from build123d import *

# Parameters (mm, degrees)
PICOVER_DEPTH                       = 40
PICOVER_DEPTH_BACK                  = 2
SKETCH1_W                           = 139.991389113
SKETCH1_H                           = 97.393342316
SKETCH2_W                           = 96.759944342
SKETCH2_H                           = 98.11966003
OPENINGFORPI_DEPTH                  = 37
SKETCH4_W                           = 18
SKETCH4_H                           = 97.393342316
CUTAWAYSTHATDEFINESCREWPLATES_DEPTH = 30
BOSS_EXTRUDE1_DEPTH                 = 97.393342316
HOLEFORPOWERHDMIAUDIO_DEPTH         = 150
HOLEFORPOWERHDMIAUDIO_DEPTH_BACK    = 30
SKETCH6_W                           = 65.470403297
SKETCH6_H                           = 37
SKETCH7_R                           = 2.75
CUT_EXTRUDE7_DEPTH                  = 60
FILLET1_R                           = 30
FILLET2_R                           = 30
FILLET3_R                           = 30
FILLET4_R                           = 30


with BuildPart() as part:
    # Sketch1 → PiCover (new, two sides: drawn at the far end of the back side and taken through both)
    with BuildSketch(Plane(origin=(0, 0, 0), x_dir=(1, 0, 0), z_dir=(0, 1, 0)).offset(-PICOVER_DEPTH_BACK)):
        with Locations((69.995694556, 48.696671158)):
            Rectangle(SKETCH1_W, SKETCH1_H)
    extrude(amount=PICOVER_DEPTH + PICOVER_DEPTH_BACK)

    # Sketch2 → OpeningForPi (cut)
    with BuildSketch(Plane(origin=(0, 40, 0), x_dir=(1, 0, 0), z_dir=(0, 1, 0))):
        with Locations((70.044375284, 48.333512301)):
            Rectangle(SKETCH2_W, SKETCH2_H)
    extrude(amount=-OPENINGFORPI_DEPTH, mode=Mode.SUBTRACT)

    # Sketch4 → CutAwaysThatDefineScrewPlates (cut)
    with BuildSketch(Plane.XZ.offset(2)):
        with Locations((130.991389113, -48.696671158)):
            Rectangle(SKETCH4_W, SKETCH4_H)
        with Locations((9, -48.696671158)):
            Rectangle(SKETCH4_W, SKETCH4_H)
    extrude(amount=-CUTAWAYSTHATDEFINESCREWPLATES_DEPTH, mode=Mode.SUBTRACT)

    # Sketch11 → Boss-Extrude1 (add)
    with BuildSketch(Plane.XY):
        Polygon((0, 28), (18, 28), (18, -2), align=None)
        Polygon((139.991389113, 28), (121.991389113, 28), (121.991389113, -2), align=None)
    extrude(amount=-BOSS_EXTRUDE1_DEPTH)

    # Sketch6 → HoleForPowerHDMIAudio (cut, two sides: drawn at the far end of the back side and taken through both)
    with BuildSketch(Plane(origin=(21.664403113, 0, 0), x_dir=(0, 0, -1), z_dir=(1, 0, 0)).offset(-HOLEFORPOWERHDMIAUDIO_DEPTH_BACK)):
        with Locations((47.655232797, 21.5)):
            Rectangle(SKETCH6_W, SKETCH6_H)
    extrude(amount=HOLEFORPOWERHDMIAUDIO_DEPTH + HOLEFORPOWERHDMIAUDIO_DEPTH_BACK, mode=Mode.SUBTRACT)

    # Sketch7 → Cut-Extrude7 (cut)
    with BuildSketch(Plane(origin=(0, 40, 0), x_dir=(1, 0, 0), z_dir=(0, 1, 0))):
        with Locations(Location((6.934452889, 8.128892452, 0), (0, 0, 270))):
            Circle(SKETCH7_R)
        with Locations(Location((6.934452889, 91.275593332, 0), (0, 0, 270))):
            Circle(SKETCH7_R)
        with Locations(Location((130.288718206, 89.274198859, 0), (0, 0, 270))):
            Circle(SKETCH7_R)
        with Locations(Location((129.818664093, 7.39541328, 0), (0, 0, 270))):
            Circle(SKETCH7_R)
    extrude(amount=-CUT_EXTRUDE7_DEPTH, mode=Mode.SUBTRACT)

    # Fillet1
    fillet1_edges = [part.edges().sort_by_distance(p)[0] for p in [
        (21.664403113, 3, -88.891888381),
    ]]
    fillet(fillet1_edges, radius=FILLET1_R)

    # Fillet2
    fillet2_edges = [part.edges().sort_by_distance(p)[0] for p in [
        (118.424347455, 3, -88.891888381),
    ]]
    fillet(fillet2_edges, radius=FILLET2_R)

    # Fillet3
    fillet3_edges = [part.edges().sort_by_distance(p)[0] for p in [
        (21.664403113, 3, -7.460015574),
    ]]
    fillet(fillet3_edges, radius=FILLET3_R)

    # Fillet4
    fillet4_edges = [part.edges().sort_by_distance(p)[0] for p in [
        (118.424347455, 3, -7.460015574),
    ]]
    fillet(fillet4_edges, radius=FILLET4_R)


solid = part.part
Build history of the part. All positions in model axes, mm. A direction names the side the tool comes from. Round coordinates to 2 decimals unless told otherwise and drop trailing zeros. Write each loop counter-clockwise with the first axis right and the second up, starting at its lowest first coordinate (ties: lowest second). Pieces come first, ordered by that corner, then holes. Notation, with made-up numbers: M 57,15 L 76,15 A21 ccw 76,47 Z; hole C 9.5,-35 d4. An arc over 180 degrees is marked long. Answer as a JSON object with one key per item and string values. Group by question number.
(1) Flat gauge pins, fed straight in: pin 1 (6 mm diameter, centred on y = 26.5, z = -85.5, fed in from -X); pin 2 (1 mm diameter, centred on x = 57, z = -46, fed in from +Y); pin 3 (6.5 mm diameter, centred on x = 129.82, z = -7.4, fed in from -Y); pin 4 (6.5 mm diameter, centred on x = 130.29, z = -89.27, fed in from -Y). Where does each tip first touch, or does it go through?
(2) Drill centre lines: L1, parallel to Z at x = 7, y = 22; L2, parallel to X at y = 32.5, z = -84; L3, parallel to Z at x = 17, y = 24. Where is each one in solid material? Low to high.
(3) Cut at A-A (y = 26). Give the cut face in (x, z).
(4) Mould opens along X. For faces 5 (the flat face through (124.865, 2.79, -48.015)), 6 (the flat face through (127, 40, -89)), 7 (the flat face through (118.424, 37, -89)) say: pulls with the +X half, pulls with the -X half, needs draft (parallel to the pull), parting line crosses it, or undercut.
(5) Cut at B-B (x = 92). Give the cut face in (y, z), and give its area (3 significant figures).
(6) Cut at D-D (x = 59.5). Give the cut face in (y, z).
(7) Which spindle directions (+Z, -Z, +X, -X, +Y, -Y) get a long thin tool onto all of the face, cutting with end or side? Do faces 1 (the cylindrical face through (127.134, 27.192, -7.992)), 2 (the cylindrical face through (30.22, 12.02, -7.56)), 3 (the flat face through (69, 3, -48)), 4 (the flat face through (14, 21, -80.39)). Say none if no direction does.
(8) Cut at C-C (z = -26). Give the cut face in (x, y), and give its area (3 significant figures).
Responses:
{
 "1": {"pin 1": "stops at x = 0", "pin 2": "stops at y = 3", "pin 3": "stops at y = 5.63", "pin 4": "stops at y = 6.41"},
 "2": {"L1": "z = -97.39 to -94.02, -88.53 to -80.39, -14.92 to -10.88, -5.38 to 0", "L2": "x = 0 to 21.67, 118.42 to 139.99", "L3": "z = -97.39 to -80.39, -14.92 to 0"},
 "3": {"outline": "M 1.2,-97.39 L 22.49,-97.39 L 22.49,-80.39 L 1.2,-80.39 Z; M 1.2,-14.92 L 22.49,-14.92 L 22.49,0 L 1.2,0 Z; M 117.6,-97.39 L 138.79,-97.39 L 138.79,-80.39 L 117.6,-80.39 Z; M 117.6,-14.92 L 138.79,-14.92 L 138.79,0 L 117.6,0 Z; hole C 6.93,-91.28 d5.5; hole C 6.93,-8.13 d5.5; hole C 129.82,-7.4 d5.5; hole C 130.29,-89.27 d5.5"},
 "4": {"face 5": "pulls with the +X half", "face 6": "needs draft", "face 7": "undercut"},
 "5": {"outline": "M -2,-97.39 L 3.21,-97.39 L 3.21,-80.39 L 3,-80.39 L 3,-14.92 L 3.21,-14.92 L 3.21,0 L -2,0 Z", "area": "494 mm2"},
 "6": {"outline": "M -2,-97.39 L 3,-97.39 L 3,0 L -2,0 Z"},
 "7": {"face 1": "+Y, -Y", "face 2": "+Z, -Z, +Y", "face 3": "+Y", "face 4": "+X, -X, +Y"},
 "8": {"outline": "M 15,3 L 18,-2 L 121.99,-2 L 124.99,3 Z", "area": "535 mm2"}
}
